For this review, take the finished solid that the model builds, in its own axes (mm). A direction names the side the tool comes from. Round coordinates to 2 decimals unless told otherwise and drop trailing zeros. Loops run counter-clockwise (first coordinate to the right, second up) from the corner with the lowest first, then second, coordinate; pieces in that order, holes last. Notation, with made-up numbers: (78.25, 71) -> (129.25, 71) arc R34 ccw to (129.25, 109) -> close; hole circle Ø9 at (13.25, 28). An arc over 180 degrees is marked (long way). One line per question, with ' | ' between items. Start each with the question number.
1. Consider section D-D (y = 52.7). Write out the cut boundary in (x, z) (3 decimals), and give its area (3 significant figures).
2. Draft analysis for pull direction Z (two halves, no side actions). For faces 1 (the face through (21, -24, 0)), 2 (the face through (-12.849, 56.075, 39.665)), 3 (the face through (0, 53, 38.1)), state which applies: pulls with the +Z half, pulls with the -Z half, needs draft (parallel to the pull), parting line crosses it, or undercut.
3. Consider section B-B (y = 0). Write out the cut boundary in (x, z).
4. Consider section C-C (z = 36). Write out the cut boundary in (x, y), and give its area (3 significant figures).
5. For faces 4 (the face through (0, 53, 12.7)), 5 (the face through (0, 65.4, 11)), 6 (the face through (4.036, 30.736, 0.986)), 7 (the face through (-25.4, 36, 26)), 8 (the face through (-12.7, 0, 26)), list the 3-axis set-ups (+Z, -Z, +X, -X, +Y, -Y) from which the entire face can be reached by the end or side of a thin tool; tool diameter is ignored.
6. Consider section A-A (x = 0). Write out the cut boundary in (y, z) (3 decimals), and give its area (3 significant figures).
7. Wall thickness on line 1 along X through (y, z) = (52.7, 40.3); line 2 along Z through (x, y) = (8.5, 60.5) (3 decimals); line 3 along Y through (x, z) = (-12, 39): over which ranges is each line inside the solid? List them lowest first.
8. For pin 1 Ø3 at (y, z) = (-24, 10.5) entering from -X; pin 2 Ø1.5 at (x, z) = (-25.5, 22) entering from -Y; pin 3 Ø6 at (x, z) = (-5.5, 5.5) entering from -Y, all flat-tipped, find the tip position at first contact; note any pin that passes through.
Autodesk Inventor part; units mm, degrees
ref_plane "XZ Plane" through (0, 0, 0) normal (0, 1, 0) x (-1, 0, 0)
ref_plane "XY Plane" through (0, 0, 0) normal (0, 0, 1) x (1, 0, 0)
sketch "Sketch1" plane through (0, 0, 0) normal (0, 0, 1) x (1, 0, 0)
  circle A0 centre (0, 0) radius 40
  dimension "d0" = 80
extrude "Extrusion1" add sketch "Sketch1" along normal blind 50.8
sketch "Sketch2" plane through (0, 0, 0) normal (0, 0, -1) x (-1, 0, 0)
  circle A0 centre (0, 0) radius 31
  circle A1 centre (0, 0) radius 24
  dimension "d3" = 62
  dimension "d4" = 48
extrude "Extrusion2" cut sketch "Sketch2" against normal blind 2
sketch "Sketch3" plane through (0, 0, 0) normal (0, 0, -1) x (-1, 0, 0)
  circle A0 centre (0, 0) radius 3.175
  dimension "d25" = 6.35
extrude "Extrusion3" cut sketch "Sketch3" against normal through all
sketch "Sketch4" plane through (0, 0, 50.8) normal (0, 0, 1) x (1, 0, 0)
  line L0 (-12.7, -6.35) -> (12.7, -6.35)
  line L1 (12.7, -6.35) -> (12.7, 6.35)
  line L2 (12.7, 6.35) -> (-12.7, 6.35)
  line L3 (-12.7, 6.35) -> (-12.7, -6.35)
  line L4 (-12.7, -6.35) -> (12.7, 6.35) construction
  line L5 (12.7, -6.35) -> (-12.7, 6.35) construction
  point P0 (0, 0)
  dimension "d28" = 25.4
  dimension "d29" = 12.7
extrude "Extrusion4" cut sketch "Sketch4" against normal through all
sketch "Sketch6" plane through (0, 0, 0) normal (1, 0, 0) x (0, 1, 0)
  line L0 (40, 0) -> (40, 50.8) construction
  line L1 (40, 25.4) -> (-40, 25.4) construction
  line L2 (-40, 0) -> (-40, 50.8) construction
  line L3 (40, 9.525) -> (65.4, 9.525)
  line L4 (65.4, 9.525) -> (65.4, 25.4)
  line L5 (40, 25.4) -> (27.3, 25.4)
  line L6 (27.3, 9.525) -> (40, 9.525)
  line L7 (27.3, 25.4) -> (27.3, 9.525)
  line L8 (40, 41.275) -> (65.4, 41.275)
  line L9 (65.4, 41.275) -> (65.4, 25.4)
  line L10 (27.3, 41.275) -> (40, 41.275)
  line L11 (27.3, 25.4) -> (27.3, 41.275)
  point P0 (0, 0)
  dimension "d34" = 25.4
  dimension "d35" = 12.7
  dimension "d36" = 15.875
extrude "Extrusion5" add sketch "Sketch6" along normal mid plane 50.8
sketch "Sketch8" plane through (-25.4, 65.4, 41.275) normal (0, 1, 0) x (1, 0, 0)
  line L0 (0, 31.75) -> (50.8, 31.75)
  line L1 (0, 3.175) -> (50.8, 3.175)
  line L2 (50.8, 3.175) -> (50.8, 28.575)
  line L3 (50.8, 28.575) -> (0, 28.575)
  line L4 (0, 28.575) -> (0, 3.175)
  line L5 (0, 3.175) -> (50.8, 28.575) construction
  line L6 (50.8, 3.175) -> (0, 28.575) construction
  point P0 (25.4, 41.275)
  point P1 (25.4, 15.875)
  dimension "d43" = 15.875
  dimension "d44" = 25.4
extrude "Extrusion7" cut sketch "Sketch8" against normal blind 25.4
sketch "Sketch9" plane through (0, 0, 41.275) normal (0, 0, 1) x (1, 0, 0)
  line L0 (-25.4, 65.4) -> (25.4, 65.4)
  line L1 (0, 86.48) -> (0, -61.08)
  point P0 (0, 0)
  point P1 (-12.7, 52.7)
  point P2 (12.7, 52.7)
  dimension "d47" = 12.7
  dimension "d48" = 12.7
  dimension "d49" = 12.7
  dimension "d50" = 12.7
hole "Hole1" at (-12.7, 52.7, 41.275) at (12.7, 52.7, 41.275) direction (0, 0, -1) diameter 6.7564 end through all
equation "\"d0\" = mountOuterDiameter"
equation "\"d3\" = ringOuterDiam + ringDiamGap"
equation "\"d4\" = ringInnerDiam - ringDiamGap"
equation "\"ringOuterDiam\" = 60"
equation "\"ringInnerDiam\" = 50"
equation "\"ringThickness\" = 1.5"
equation "\"ringDiamGap\" = 2"
equation "\"mountOuterDiameter\" = 80"
properties part number "MountV05"
Answer block:
1) outline: (-25.4, 9.525) -> (-16.078, 9.525) -> (-16.078, 12.7) -> (-25.4, 12.7) -> close; (-25.4, 38.1) -> (-16.078, 38.1) -> (-16.078, 41.275) -> (-25.4, 41.275) -> close; (-9.322, 9.525) -> (9.322, 9.525) -> (9.322, 12.7) -> (-9.322, 12.7) -> close; (-9.322, 38.1) -> (9.322, 38.1) -> (9.322, 41.275) -> (-9.322, 41.275) -> close; (16.078, 9.525) -> (25.4, 9.525) -> (25.4, 12.7) -> (16.078, 12.7) -> close; (16.078, 38.1) -> (25.4, 38.1) -> (25.4, 41.275) -> (16.078, 41.275) -> close | area: 237 mm2
2) face 1: pulls with the -Z half | face 2: needs draft | face 3: undercut
3) outline: (-40, 0) -> (-31, 0) -> (-31, 2) -> (-24, 2) -> (-24, 0) -> (-12.7, 0) -> (-12.7, 50.8) -> (-40, 50.8) -> close; (12.7, 0) -> (24, 0) -> (24, 2) -> (31, 2) -> (31, 0) -> (40, 0) -> (40, 50.8) -> (12.7, 50.8) -> close
4) outline: (-25.4, 30.9) arc R40 ccw (long way) to (25.4, 30.9) -> (25.4, 40) -> (-25.4, 40) -> close; hole (-12.7, -6.35) -> (12.7, -6.35) -> (12.7, 6.35) -> (-12.7, 6.35) -> close | area: 4,850 mm2
5) face 4: +X, -X, +Y | face 5: +Z, -Z, +X, -X, +Y | face 6: -Z | face 7: +Z, -Z, -X, +Y | face 8: +Z, -Z
6) outline: (-40, 0) -> (-31, 0) -> (-31, 2) -> (-24, 2) -> (-24, 0) -> (-6.35, 0) -> (-6.35, 50.8) -> (-40, 50.8) -> close; (6.35, 0) -> (24, 0) -> (24, 2) -> (31, 2) -> (31, 0) -> (40, 0) -> (40, 9.525) -> (65.4, 9.525) -> (65.4, 12.7) -> (40, 12.7) -> (40, 38.1) -> (65.4, 38.1) -> (65.4, 41.275) -> (40, 41.275) -> (40, 50.8) -> (6.35, 50.8) -> close | area: 3,550 mm2
7) line 1: x = -25.4 to -16.08, -9.32 to 9.32, 16.08 to 25.4 | line 2: z = 9.525 to 12.7, 38.1 to 41.275 | line 3: y = -38.16 to -6.35, 6.35 to 49.4, 56 to 65.4
8) pin 1: stops at x = -33.07 | pin 2: stops at y = -31.42 | pin 3: stops at y = -39.92
